The model under review builds one solid part; all positions refer to its coordinate system, in mm. A direction names the side the tool comes from. Coordinates: 2 decimals unless noted, no trailing zeros. Order: outer loops, then holes, each group sorted by start corner. A loop starts at its lowest first (then second) coordinate and runs counter-clockwise, first axis right, second up. Notation, with made-up numbers: (68, -25.75) - (91, -25.75) arc R12 ccw to (91, -18.75) - close; hole circle Ø10 at (81.5, 29). An arc over 180 degrees is marked (long way). Answer in a Markdown table with one row per item.
```python
from build123d import *

# Parameters (mm, degrees)
F0_R     = 2.5
F1_DEPTH = 8
F3_R     = 12
F4_R     = 5
F5_R     = 5


with BuildPart() as f1:
    # F0 (on Top) → F1 (new body)
    with BuildSketch(Plane.XY):
        with BuildLine():
            Line((0, -35), (7.2830180969, -35))
            ThreePointArc((7.2830180969, -35), (77.2966007948, -66.3705025512), (131.4247694765, -12))
            Line((131.4247694765, -12), (145, -12))
            Line((145, -12), (145, 28))
            Line((145, 28), (126.4186453774, 28))
            ThreePointArc((126.4186453774, 28), (65, 67.5), (3.5813546226, 28))
            Line((3.5813546226, 28), (0, 28))
            Line((0, 28), (0, 0))
            Line((0, 0), (0, -35))
        make_face()
        with Locations((137, -4)):
            Circle(F0_R, mode=Mode.SUBTRACT)
        with Locations((137, 20)):
            Circle(F0_R, mode=Mode.SUBTRACT)
    extrude(amount=F1_DEPTH)

    # F2: F1 across face


with BuildPart() as f1_1:
    add(f1.part)
    add(f1.part.mirror(Plane(origin=(0, -3.5, 4), x_dir=(0, -1, 0), z_dir=(-1, 0, 0))))

    # F3
    f3_edges = [f1_1.edges().sort_by_distance(p)[0] for p in [
        (7.283018, -35, 4),
        (-7.283018, -35, 4),
    ]]
    fillet(f3_edges, radius=F3_R)

    # F4
    f4_edges = [f1_1.edges().sort_by_distance(p)[0] for p in [
        (131.424769, -12, 4),
        (126.418645, 28, 4),
        (-126.418645, 28, 4),
        (-131.424769, -12, 4),
    ]]
    fillet(f4_edges, radius=F4_R)

    # F5
    f5_edges = [f1_1.edges().sort_by_distance(p)[0] for p in [
        (-3.581355, 28, 4),
        (3.581355, 28, 4),
    ]]
    fillet(f5_edges, radius=F5_R)


solid = f1_1.part
```
Item 1: Mouldability with a two-part tool opening along Y and no side actions: class faces 1 (the face through (66.04, 67.49, 3.94)), 2 (the face through (6.236, -36.261, 4.056)), 3 (the face through (145, 8, 4)), 4 (the face through (-139.385, -3.249, 3.944)) as +Y half, -Y half, draft (parallel to the pull), parting line (faces both ways), or undercut.
Check values:
| item | result |
|---|---|
| face 1 | +Y half |
| face 2 | -Y half |
| face 3 | draft |
| face 4 | undercut |
Item 2: We need section A-A, the plane z = 2.5. Write out the cut boundary in (x, y), then the cut area to 3 significant figures.
Check values:
| item | result |
|---|---|
| outline | (-145, -12) - (-135.48, -12) arc R5 cw to (-130.62, -15.83) arc R67.5 ccw to (-10.56, -39.91) arc R12 cw to (-0.88, -35) - (0.88, -35) arc R12 cw to (10.56, -39.91) arc R67.5 ccw to (130.62, -15.83) arc R5 cw to (135.48, -12) - (145, -12) - (145, 28) - (129.55, 28) arc R5 cw to (125.1, 30.72) arc R67.5 ccw to (4.9, 30.72) arc R5 cw to (0.45, 28) - (-0.45, 28) arc R5 cw to (-4.9, 30.72) arc R67.5 ccw to (-125.1, 30.72) arc R5 cw to (-129.55, 28) - (-145, 28) - close; hole circle Ø5 at (-137, -4); hole circle Ø5 at (-137, 20); hole circle Ø5 at (137, -4); hole circle Ø5 at (137, 20) |
| area | 29,700 mm^2 |
Item 3: We need section B-B, the plane y = 56. Write out the cut boundary in (x, z).
Check values:
| item | result |
|---|---|
| outline | (-102.69, 0) - (-27.31, 0) - (-27.31, 8) - (-102.69, 8) - close; (27.31, 0) - (102.69, 0) - (102.69, 8) - (27.31, 8) - close |
Item 4: We need section C-C, the plane x = -25.5. Write out the cut boundary in (y, z), then the cut area to 3 significant figures.
Check values:
| item | result |
|---|---|
| outline | (-54.74, 0) - (54.74, 0) - (54.74, 8) - (-54.74, 8) - close |
| area | 876 mm^2 |
Item 5: Tool access review of faces 5 (the face through (140, -12, 4)), 6 (the face through (-6.236, -36.261, 4.056)), 7 (the face through (137, 28, 4)), 8 (the face through (-132.35, -13.1, 4.06)), 9 (the face through (-66.04, 67.49, 3.94)): name each direction out of +Z, -Z, +X, -X, +Y, -Y from which nothing blocks a thin tool from reaching the whole face with its end or side.
Check values:
| item | result |
|---|---|
| face 5 | +Z, -Z, +X, -Y |
| face 6 | +Z, -Z, -Y |
| face 7 | +Z, -Z, +X, +Y |
| face 8 | +Z, -Z, -X, -Y |
| face 9 | +Z, -Z, +Y |
Item 6: We need section D-D, the plane y = -31. Write out the cut boundary in (x, z).
Check values:
| item | result |
|---|---|
| outline | (-124.96, 0) - (124.96, 0) - (124.96, 8) - (-124.96, 8) - close |
Item 7: Clearance check with flat-ended pins moving along their axes: pin 1 Ø3 at (y, z) = (30.5, 6.5) entering from -X; pin 2 Ø1.5 at (x, z) = (-22, 3) entering from +Y; pin 3 Ø1.9 at (x, z) = (0, 5) entering from -Y; pin 4 Ø6 at (x, y) = (-137, -4) entering from -Z. State where each tip first meets the part, or that it passes through.
Check values:
| item | result |
|---|---|
| pin 1 | x = -126.55 |
| pin 2 | y = 52.64 |
| pin 3 | y = -35 |
| pin 4 | z = 0 |
Item 8: To check wall thickness, follow line 1 (Y direction, x = 137, z = 1.75); line 2 (X direction, y = -62, z = 4.25); line 3 (X direction, y = 38.5, z = 2.5). State the ranges of each line that lie inside material, in increasing order. Write a range as from..to.
Check values:
| item | result |
|---|---|
| line 1 | -12..-6.5, -1.5..17.5, 22.5..28 |
| line 2 | -91.69..-38.31, 38.31..91.69 |
| line 3 | -120.44..-9.56, 9.56..120.44 |
